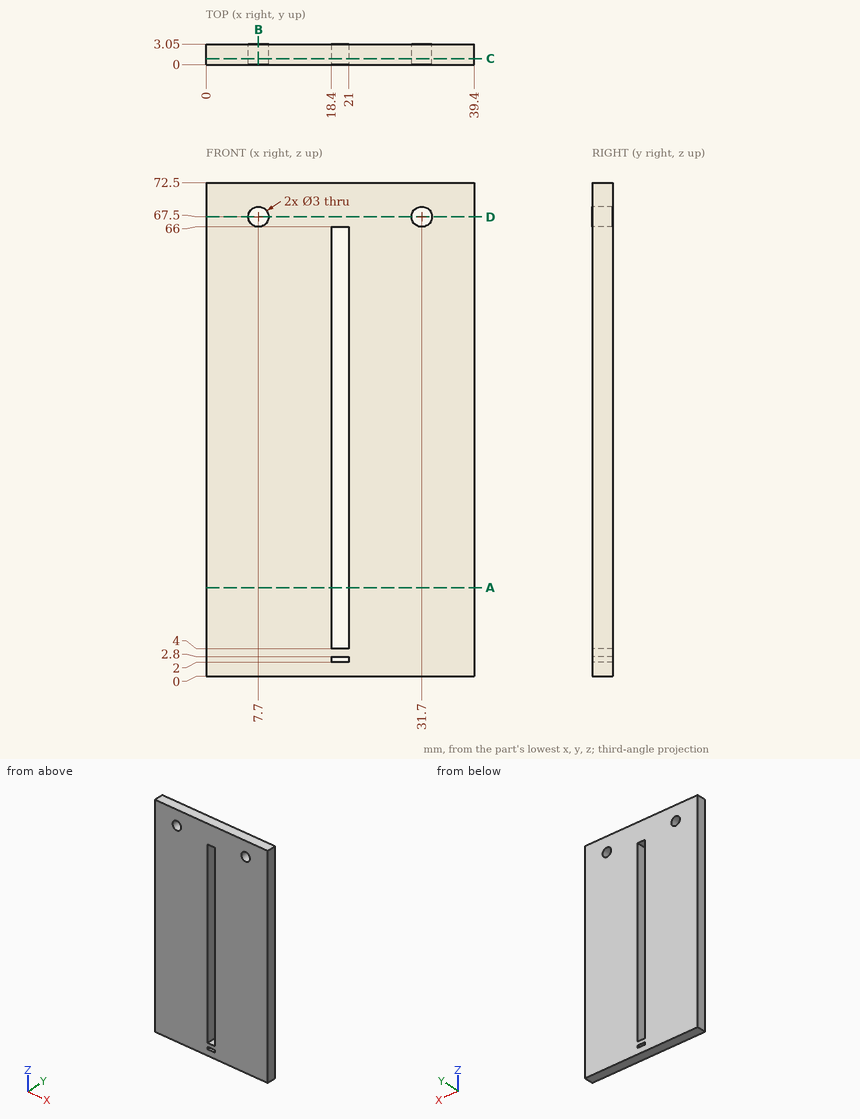
The drawing under review shows one solid part. Ordinate dimensions are in mm from its lowest x, y, z. Coordinates: 2 decimals unless noted, no trailing zeros. Write each loop counter-clockwise with the first axis right and the second up, starting at its lowest first coordinate (ties: lowest second). Pieces come first, ordered by that corner, then holes. Notation, with made-up numbers: (-16.75, 56) - (-12.75, 56) arc R20 cw to (-12.75, 79) - close; hole circle Ø6 at (-25, 67). An arc over 180 degrees is marked (long way). Put each result on its own line as item: value.
1. Wall thickness on probe 1 along X at (y, z) = (2.15, 67.5); probe 2 along Z at (x, y) = (31.7, 1.4); probe 3 along X at (y, z) = (0.2, 49): over which ranges is each line inside the solid? List them lowest first.
Values found:
probe 1: 0 to 6.2, 9.2 to 30.2, 33.2 to 39.4
probe 2: 0 to 66, 69 to 72.5
probe 3: 0 to 18.4, 21 to 39.4
2. Add section A-A, the plane z = 13. Give the boundary of the cut face in (x, y), then the cut area to 3 significant figures.
Values found:
outline: (0, 0) - (18.4, 0) - (18.4, 3.05) - (0, 3.05) - close; (21, 0) - (39.4, 0) - (39.4, 3.05) - (21, 3.05) - close
area: 112 mm²
3. Add section B-B, the plane x = 7.7. Give the boundary of the cut face in (y, z), then the cut area to 3 significant figures.
Values found:
outline: (0, 0) - (3.05, 0) - (3.05, 66) - (0, 66) - close; (0, 69) - (3.05, 69) - (3.05, 72.5) - (0, 72.5) - close
area: 212 mm²
4. Add section C-C, the plane y = 0.9. Give the boundary of the cut face in (x, z).
Values found:
outline: (0, 0) - (39.4, 0) - (39.4, 72.5) - (0, 72.5) - close; hole circle Ø3 at (7.7, 67.5); hole (18.4, 2) - (21, 2) - (21, 2.8) - (18.4, 2.8) - close; hole (18.4, 4) - (21, 4) - (21, 66) - (18.4, 66) - close; hole circle Ø3 at (31.7, 67.5)
5. Add section D-D, the plane z = 67.5. Give the boundary of the cut face in (x, y), then the cut area to 3 significant figures.
Values found:
outline: (0, 0) - (6.2, 0) - (6.2, 3.05) - (0, 3.05) - close; (9.2, 0) - (30.2, 0) - (30.2, 3.05) - (9.2, 3.05) - close; (33.2, 0) - (39.4, 0) - (39.4, 3.05) - (33.2, 3.05) - close
area: 102 mm²
